Part model, mm, in its own coordinate system. A direction names the side the tool comes from. Round coordinates to 2 decimals unless told otherwise and drop trailing zeros. Write each loop counter-clockwise with the first axis right and the second up, starting at its lowest first coordinate (ties: lowest second). Pieces come first, ordered by that corner, then holes. Notation, with made-up numbers: M 34,16 L 66,16 A15 cw 66,23 Z; hole C 52,-15.5 d2. An arc over 180 degrees is marked long. Use one line per item in the form item = value. Start each with the question number.
Item 1: Cut at B-B, the plane y = -3.5. Give the cut face in (x, z).
Item 2: Flat gauge pins, fed straight in: pin 1 Ø6 at (x, y) = (-2, 3) entering from +Z; pin 2 Ø1 at (x, y) = (-1.5, 14.5) entering from +Z. Where does each tip first touch, or does it go through?
Item 3: Probe L1, parallel to Y at x = 1.75, z = 18; L2, parallel to X at y = 8, z = 33; L3, parallel to Y at x = -1.75, z = 22. List the from-to ranges inside material, lowest first.
Item 4: Cut at C-C, the plane x = 2.25. Give the cut face in (y, z).
Item 5: Cut at A-A, the plane z = 13.5. Give the cut face in (x, y), then the cut area to 3 significant figures.
Item 6: Which spindle directions (+Z, -Z, +X, -X, +Y, -Y) get a long thin tool onto all of the face, cutting with end or side? Do faces 1 (the face through (-7.938, 2, 12)), 2 (the face through (0, -13, 21.401)), 3 (the face through (4.762, 7, 15)). Say none if no direction does.
Item 7: Cut at D-D, the plane z = 37.5. Give the cut face in (x, y), then the cut area to 3 significant figures.
Item 8: Mould opens along Y. For faces 4 (the face through (0, 19.869, 16)), 5 (the face through (4.762, 15, 19)), 6 (the face through (0, -15.056, 7)), 7 (the face through (0, -6, 27.751)) say: +Y half, -Y half, draft (parallel to the pull), parting line (faces both ways), or undercut.
from build123d import *

# Parameters (mm, degrees)
F0_W      = 34.925
F0_H      = 47.625
F1_DEPTH  = 7.9375
F3_DEPTH  = 12.7
F4_W      = 9.525
F4_H      = 3.175
F5_DEPTH  = 44.45
F6_W      = 9.525
F6_H      = 6.35
F7_DEPTH  = 38.1
F8_W      = 9.525
F8_H      = 6.35
F9_DEPTH  = 31.75
F10_W     = 9.525
F10_H     = 3.175
F11_DEPTH = 25.4


with BuildPart() as f1:
    # F0 (on Right) → F1 (new body, symmetric)
    with BuildSketch(Plane.YZ):
        with Locations((2.406316, 16.638194)):
            Rectangle(F0_W, F0_H)
    extrude(amount=F1_DEPTH, both=True)

    # F2 (on Right) → F3 (cut, symmetric)
    with BuildSketch(Plane.YZ):
        Polygon((-15.056184, 46.800694), (-15.056184, 21.400694), (-8.706184, 21.400694), (-8.706184, 27.750694), (0.818816, 27.750694), (0.818816, 34.100694), (10.343816, 34.100694), (10.343816, 40.450694), (19.868816, 40.450694), (19.868816, 46.800694), align=None)
    extrude(amount=F3_DEPTH, both=True, mode=Mode.SUBTRACT)

    # F4 (on face) → F5 (cut)
    with BuildSketch(Plane.XY.offset(40.450694)):
        with Locations((0, 15.106316)):
            Rectangle(F4_W, F4_H)
    extrude(amount=-F5_DEPTH, mode=Mode.SUBTRACT)

    # F6 (on face) → F7 (cut)
    with BuildSketch(Plane.XY.offset(34.100694)):
        with Locations((0, 7.168816)):
            Rectangle(F6_W, F6_H)
    extrude(amount=-F7_DEPTH, mode=Mode.SUBTRACT)

    # F8 (on face) → F9 (cut)
    with BuildSketch(Plane.XY.offset(27.750694)):
        with Locations((0, -2.356184)):
            Rectangle(F8_W, F8_H)
    extrude(amount=-F9_DEPTH, mode=Mode.SUBTRACT)

    # F10 (on face) → F11 (cut)
    with BuildSketch(Plane.XY.offset(21.400694)):
        with Locations((0, -10.293684)):
            Rectangle(F10_W, F10_H)
    extrude(amount=-F11_DEPTH, mode=Mode.SUBTRACT)


solid = f1.part
Model answer:
q1.outline = M -7.94,-7.17 L 7.94,-7.17 L 7.94,27.75 L 4.76,27.75 L 4.76,-4 L -4.76,-4 L -4.76,27.75 L -7.94,27.75 Z
q2.pin_1 = 34.1
q2.pin_2 = -4
q3.L1 = -15.06 to -11.88, -8.71 to -5.53, 0.82 to 3.99, 10.34 to 13.52, 16.69 to 19.87
q3.L2 = -7.94 to -4.76, 4.76 to 7.94
q3.L3 = -8.71 to -5.53, 0.82 to 3.99, 10.34 to 13.52, 16.69 to 19.87
q4.outline = M -15.06,-7.17 L 19.87,-7.17 L 19.87,40.45 L 16.69,40.45 L 16.69,-4 L 13.52,-4 L 13.52,40.45 L 10.34,40.45 L 10.34,-4 L 3.99,-4 L 3.99,34.1 L 0.82,34.1 L 0.82,-4 L -5.53,-4 L -5.53,27.75 L -8.71,27.75 L -8.71,-4 L -11.88,-4 L -11.88,21.4 L -15.06,21.4 Z
q5.outline = M -7.94,-15.06 L 7.94,-15.06 L 7.94,19.87 L -7.94,19.87 Z; hole M -4.76,-11.88 L 4.76,-11.88 L 4.76,-8.71 L -4.76,-8.71 Z; hole M -4.76,-5.53 L 4.76,-5.53 L 4.76,0.82 L -4.76,0.82 Z; hole M -4.76,3.99 L 4.76,3.99 L 4.76,10.34 L -4.76,10.34 Z; hole M -4.76,13.52 L 4.76,13.52 L 4.76,16.69 L -4.76,16.69 Z
q5.area = 373 mm²
q6.face_1 = +Z, -Z, -X, +Y, -Y
q6.face_2 = +Z, +X, -X, -Y
q6.face_3 = +Z
q7.outline = M -7.94,10.34 L 7.94,10.34 L 7.94,19.87 L -7.94,19.87 Z; hole M -4.76,13.52 L 4.76,13.52 L 4.76,16.69 L -4.76,16.69 Z
q7.area = 121 mm²
q8.face_4 = +Y half
q8.face_5 = undercut
q8.face_6 = -Y half
q8.face_7 = draft
